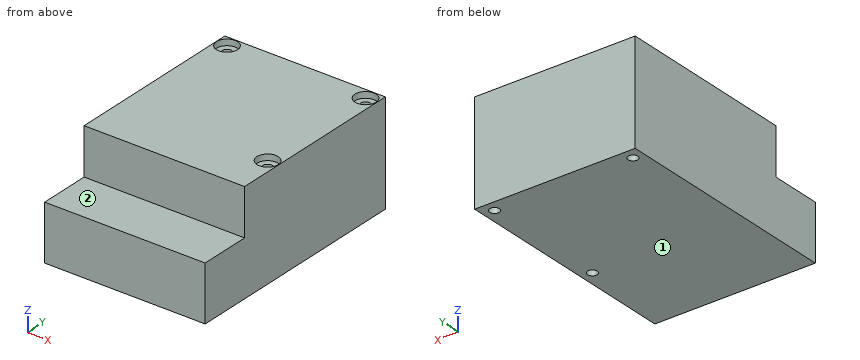
from build123d import *

# Parameters (mm, degrees)
SKETCH_1_W                   = 110
SKETCH_1_H                   = 160
EXTRUDE_1_DEPTH              = 70
SKETCH_2_W                   = 110
SKETCH_2_H                   = 20
CUT_EXTRUDE_1_DEPTH          = 35
SKETCH_9_W                   = 110
SKETCH_9_H                   = 12
CUT_EXTRUDE_2_DEPTH          = 35
HOLE_WIZARD_M6_1_D           = 6.6
HOLE_WIZARD_M6_1_CBORE_D     = 14.55
HOLE_WIZARD_M6_1_CBORE_DEPTH = 4.15


with BuildPart() as part:
    # 草图1 → 凸台-拉伸1 (new body)
    with BuildSketch(Plane.XY):
        Rectangle(SKETCH_1_W, SKETCH_1_H)
    extrude(amount=EXTRUDE_1_DEPTH)

    # 草图2 → 切除-拉伸1 (cut)
    with BuildSketch(Plane.XZ.offset(80)):
        with Locations((0, 60)):
            Rectangle(SKETCH_2_W, SKETCH_2_H)
    extrude(amount=-CUT_EXTRUDE_1_DEPTH, mode=Mode.SUBTRACT)

    # 草图9 → 切除-拉伸2 (cut)
    with BuildSketch(Plane.XZ.offset(80)):
        with Locations((0, 44)):
            Rectangle(SKETCH_9_W, SKETCH_9_H)
    extrude(amount=-CUT_EXTRUDE_2_DEPTH, mode=Mode.SUBTRACT)

    # M6 六角头螺钉的柱形沉头孔1 (through all)
    with Locations(Plane.XY.offset(70)):
        with Locations((-47.570659981, 72.32370147), (47.366931244, 72.32370147), (47.366931244, -14.668469031)):
            CounterBoreHole(HOLE_WIZARD_M6_1_D / 2, HOLE_WIZARD_M6_1_CBORE_D / 2, HOLE_WIZARD_M6_1_CBORE_DEPTH)


solid = part.part
Verification items for the finished model (mm, model axes). Face numbers are marked on the shaded views. A direction names the side the tool comes from. Give positions to 0.01 mm unless a question says otherwise; leave off trailing zeros. Write each loop counter-clockwise with the first axis right and the second up, starting at its lowest first coordinate (ties: lowest second). Pieces come first, ordered by that corner, then holes. Notation, with made-up numbers: (76.5, 26) - (125.5, 26) arc R26 ccw to (125.5, 63) - close; hole circle Ø1 at (56, -23). An arc over 180 degrees is marked (long way). Answer as CSV lines item,"result". Start each with the question number.
1. Sectioned sample at C-C (y = -68). Record the boundary of the cut face in (x, z), then the cut area to 3 significant figures.
2. Set-up check for the marked faces 1 and 2: record each of +Z, -Z, +X, -X, +Y, -Y from which the full face is reachable in a straight line by a thin tool's end or side.
3. Thickness scan on line 1 (Y direction, x = 49, z = 60); line 2 (Y direction, x = -5, z = 46); line 3 (Z direction, x = -9.5, y = -46). Record the ranges inside material, lowest first.
4. Sectioned sample at B-B (x = 18.5). Record the boundary of the cut face in (y, z).
5. Sectioned sample at A-A (z = 45). Record the boundary of the cut face in (x, y).
6. Depth check by flat-ended pin: pin 1 (6 mm diameter, centred on x = 47.37, y = -14.67, fed in from +Z); pin 2 (7.5 mm diameter, centred on x = 49, y = -12.5, fed in from +Z). Enter the tip coordinate at first touch or a pass-through.
Derived:
1,outline,"(-55, 0) - (55, 0) - (55, 38) - (-55, 38) - close"
1,area,"4,180 mm²"
2,face 1,"-Z, +X, -X, +Y, -Y"
2,face 2,"+Z, +X, -X, -Y"
3,line 1,"-45 to -17.54, -11.8 to 69.46, 75.19 to 80"
3,line 2,"-45 to 80"
3,line 3,"0 to 38"
4,outline,"(-80, 0) - (80, 0) - (80, 70) - (-45, 70) - (-45, 38) - (-80, 38) - close"
5,outline,"(-55, -45) - (55, -45) - (55, 80) - (-55, 80) - close; hole circle Ø6.6 at (-47.57, 72.32); hole circle Ø6.6 at (47.37, -14.67); hole circle Ø6.6 at (47.37, 72.32)"
6,pin 1,"through"
6,pin 2,"z = 65.85"
